For this review, take the finished solid that the model builds, in its own axes (mm). Round coordinates to 2 decimals unless told otherwise and drop trailing zeros. Write each loop counter-clockwise with the first axis right and the second up, starting at its lowest first coordinate (ties: lowest second). Pieces come first, ordered by that corner, then holes. Notation, with made-up numbers: (43, 43.25) - (57, 43.25) arc R6 cw to (57, 48.25) - close; hole circle Ø11 at (49, 87). An arc over 180 degrees is marked (long way). One line per item, written item: value. Start each with the question number.
Q1. Mouldability with a two-part tool opening along X and no side actions: class faces 1 (the face through (-1, 0, -12)), 2 (the face through (0.07, 1.52, 5.5)), 3 (the face through (50, 1, 1)) as +X half, -X half, draft (parallel to the pull), parting line (faces both ways), or undercut.
Q2. Clearance check with a flat-ended pin moving along its axis: pin 1 Ø2.5 at (x, z) = (7, 0) entering from +Y. State where the tip first meets the part, or that it passes through.
Q3. Add section D-D on z = -7. Write out the cut boundary in (x, y), and give its area (3 significant figures).
Q4. Add section A-A on x = -31.5. Write out the cut boundary in (y, z), and give its area (3 significant figures).
Q5. For probe 1 along X at (y, z) = (2.55, -2); probe 2 along X at (y, z) = (2.75, 45), list the stretches that pass through material, from the lowest coordinate up.
Q6. Add section B-B on z = -40.5. Write out the cut boundary in (x, y).
Q7. Add section C-C on x = 0. Write out the cut boundary in (y, z).
```python
from build123d import *

# Parameters (mm, degrees)
CROQUIS1_W              = 100
CROQUIS1_H              = 100
SALIENTE_EXTRUIR1_DEPTH = 3
CROQUIS6_R              = 1.55
CORTAR_EXTRUIR4_DEPTH   = 10
CROQUIS7_R              = 1.6
CORTAR_EXTRUIR5_DEPTH   = 10
CROQUIS8_R              = 2.5
CROQUIS8_R_2            = 1.5
CORTAR_EXTRUIR6_DEPTH   = 10


with BuildPart() as part:
    # Croquis1 → Saliente-Extruir1 (new body)
    with BuildSketch(Plane(origin=(0, 0, 0), x_dir=(1, 0, 0), z_dir=(0, 1, 0))):
        Rectangle(CROQUIS1_W, CROQUIS1_H)
    extrude(amount=SALIENTE_EXTRUIR1_DEPTH)

    # Croquis6 → Cortar-Extruir4 (cut)
    with BuildSketch(Plane(origin=(0, 3, 0), x_dir=(1, 0, 0), z_dir=(0, 1, 0))):
        with Locations(Location((-44, 44, 0), (0, 0, 270))):  # turned: the seam where the file's is
            Circle(CROQUIS6_R)
        with Locations(Location((44, 44, 0), (0, 0, 270))):  # turned: the seam where the file's is
            Circle(CROQUIS6_R)
        with Locations(Location((44, -44, 0), (0, 0, 270))):  # turned: the seam where the file's is
            Circle(CROQUIS6_R)
        with Locations(Location((-44, -44, 0), (0, 0, 270))):  # turned: the seam where the file's is
            Circle(CROQUIS6_R)
    extrude(amount=-CORTAR_EXTRUIR4_DEPTH, mode=Mode.SUBTRACT)

    # Croquis7 → Cortar-Extruir5 (cut)
    with BuildSketch(Plane(origin=(0, 3, 0), x_dir=(1, 0, 0), z_dir=(0, 1, 0))):
        with Locations(Location((-31.5, 40.5, 0), (0, 0, 270))):  # turned: the seam where the file's is
            Circle(CROQUIS7_R)
        with Locations(Location((31.5, 40.5, 0), (0, 0, 270))):  # turned: the seam where the file's is
            Circle(CROQUIS7_R)
        with Locations(Location((-31.5, -40.5, 0), (0, 0, 270))):  # turned: the seam where the file's is
            Circle(CROQUIS7_R)
        with Locations(Location((31.5, -40.5, 0), (0, 0, 270))):  # turned: the seam where the file's is
            Circle(CROQUIS7_R)
    extrude(amount=-CORTAR_EXTRUIR5_DEPTH, mode=Mode.SUBTRACT)

    # Croquis8 → Cortar-Extruir6 (cut)
    with BuildSketch(Plane(origin=(0, 3, 0), x_dir=(1, 0, 0), z_dir=(0, 1, 0))):
        with Locations(Location((0, 0, 0), (0, 0, 270))):  # turned: the seam where the file's is
            Circle(CROQUIS8_R)
        with Locations(Location((0, 7, 0), (0, 0, 270))):  # turned: the seam where the file's is
            Circle(CROQUIS8_R_2)
        with Locations(Location((7, 0, 0), (0, 0, 270))):  # turned: the seam where the file's is
            Circle(CROQUIS8_R_2)
        with Locations(Location((0, -7, 0), (0, 0, 270))):  # turned: the seam where the file's is
            Circle(CROQUIS8_R_2)
        with Locations(Location((-7, 0, 0), (0, 0, 270))):  # turned: the seam where the file's is
            Circle(CROQUIS8_R_2)
    extrude(amount=-CORTAR_EXTRUIR6_DEPTH, mode=Mode.SUBTRACT)


solid = part.part
```
Result set:
1. face 1: draft
1. face 2: undercut
1. face 3: +X half
2. pin 1: passes through
3. outline: (-50, 0) - (-1.5, 0) - (-1.5, 3) - (-50, 3) - close; (1.5, 0) - (50, 0) - (50, 3) - (1.5, 3) - close
3. area: 291 mm^2
4. outline: (0, -50) - (3, -50) - (3, -42.1) - (0, -42.1) - close; (0, -38.9) - (3, -38.9) - (3, 38.9) - (0, 38.9) - close; (0, 42.1) - (3, 42.1) - (3, 50) - (0, 50) - close
4. area: 281 mm^2
5. probe 1: x = -50 to -1.5, 1.5 to 50
5. probe 2: x = -50 to -45.18, -42.82 to 42.82, 45.18 to 50
6. outline: (-50, 0) - (-33.1, 0) - (-33.1, 3) - (-50, 3) - close; (-29.9, 0) - (29.9, 0) - (29.9, 3) - (-29.9, 3) - close; (33.1, 0) - (50, 0) - (50, 3) - (33.1, 3) - close
7. outline: (0, -50) - (3, -50) - (3, -8.5) - (0, -8.5) - close; (0, -5.5) - (3, -5.5) - (3, -2.5) - (0, -2.5) - close; (0, 2.5) - (3, 2.5) - (3, 5.5) - (0, 5.5) - close; (0, 8.5) - (3, 8.5) - (3, 50) - (0, 50) - close
